Geometry: final body of the model. Coordinates: model frame, mm. A direction names the side the tool comes from. Give positions to 0.01 mm unless a question says otherwise; leave off trailing zeros. Write each loop counter-clockwise with the first axis right and the second up, starting at its lowest first coordinate (ties: lowest second). Pieces come first, ordered by that corner, then holes. Notation, with made-up numbers: (-33, 60) -> (-14, 60) arc R17 ccw to (-14, 92) -> close; hole circle Ø3 at (22, 38). An arc over 180 degrees is marked (long way). Answer in a Markdown table with one row per item. Add a question column.
from build123d import *

# Parameters (mm, degrees)
ESQUISSE3_R        = 2
ESQUISSE3_W        = 6
ESQUISSE3_H        = 6
ESQUISSE3_W_2      = 6.1
ESQUISSE3_H_2      = 6.1
ESQUISSE3_W_3      = 6.2
ESQUISSE3_H_3      = 6.2
ESQUISSE3_W_4      = 6.3
ESQUISSE3_H_4      = 6.3
BOSS_EXTRU_1_DEPTH = 6


with BuildPart() as part:
    # Esquisse3 → Boss.-Extru.1 (new body)
    with BuildSketch(Plane.XY):
        with BuildLine():
            Line((-87.161685907, 41.494801679), (-87.161685907, -2.505198321))
            Line((-87.161685907, -2.505198321), (-59.161685907, -2.505198321))
            Line((-59.161685907, -2.505198321), (-59.161685907, 41.494801679))
            ThreePointArc((-59.161685907, 41.494801679), (-73.161685907, 44.961803356), (-87.161685907, 41.494801679))
        make_face()
        with Locations((-73.161685907, 34.494801679)):
            Circle(ESQUISSE3_R, mode=Mode.SUBTRACT)
        with Locations((-73.161685907, 24.544801679)):
            Circle(ESQUISSE3_R, mode=Mode.SUBTRACT)
        with Locations((-73.161685907, 14.594801679)):
            Circle(ESQUISSE3_R, mode=Mode.SUBTRACT)
        with Locations((-73.161685907, 4.644801679)):
            Circle(ESQUISSE3_R, mode=Mode.SUBTRACT)
        with Locations((-80.161685907, 34.494801679)):
            Rectangle(ESQUISSE3_W, ESQUISSE3_H, mode=Mode.SUBTRACT)
        with Locations((-66.161685907, 34.494801679)):
            Rectangle(ESQUISSE3_W, ESQUISSE3_H, mode=Mode.SUBTRACT)
        with Locations((-80.161685907, 24.544801679)):
            Rectangle(ESQUISSE3_W_2, ESQUISSE3_H_2, mode=Mode.SUBTRACT)
        with Locations((-66.161685907, 24.544801679)):
            Rectangle(ESQUISSE3_W_2, ESQUISSE3_H_2, mode=Mode.SUBTRACT)
        with Locations((-80.161685907, 14.594801679)):
            Rectangle(ESQUISSE3_W_3, ESQUISSE3_H_3, mode=Mode.SUBTRACT)
        with Locations((-66.161685907, 14.594801679)):
            Rectangle(ESQUISSE3_W_3, ESQUISSE3_H_3, mode=Mode.SUBTRACT)
        with Locations((-80.161685907, 4.644801679)):
            Rectangle(ESQUISSE3_W_4, ESQUISSE3_H_4, mode=Mode.SUBTRACT)
        with Locations((-66.161685907, 4.644801679)):
            Rectangle(ESQUISSE3_W_4, ESQUISSE3_H_4, mode=Mode.SUBTRACT)
    extrude(amount=BOSS_EXTRU_1_DEPTH)


solid = part.part
Q1. Section B-B on y = 35. Return loops of the section in (x, z), and give its area (3 significant figures).
Q2. Section A-A on x = -66.5. Return loops of the section in (y, z), and give its area (3 significant figures).
Q3. Pull-direction query (Y, two-part tool) for faces 3 (the flat face through (-80, 17.695, 3)), 4 (the flat face through (-59.162, 19, 3)), 5 (the cylindrical face through (-72.96, 44.96, 2.96)); classes: +Y half, -Y half, draft (parallel to the pull), parting line (faces both ways), or undercut.
Q4. Contact query for flat-ended pins moving along their axis: pin 1 Ø1.5 at (x, z) = (-76, 1) entering from +Y; pin 2 Ø6 at (x, y) = (-68.5, 12.5) entering from +Z. Output: stop coordinate, or through.
Q5. Access query for faces 1 (the flat face through (-66, 21.495, 3)), 2 (the flat face through (-73, -2.505, 3)). Directions: +Z, -Z, +X, -X, +Y, -Y. A direction counts if a zero-diameter tool reaches every point of the face in a straight line with its end or side. Return the directions, or none.
Q6. Section C-C on x = -71.75. Return loops of the section in (y, z).
Q7. Section D-D on z = 3.55. Count the separate pieces of the cut face and the enclosed holes in it, and give its area (3 significant figures).
Q8. Line query: probe 1 along X at (y, z) = (4.5, 2); probe 2 along X at (y, z) = (24.5, 0.7); probe 3 along Y at (x, z) = (-68.5, 1.4). Output: solid intervals per line, ascending. Write a range as from..to.
Checks:
| question | item | result |
|---|---|---|
| 1 | outline | (-87.16, 0) -> (-83.16, 0) -> (-83.16, 6) -> (-87.16, 6) -> close; (-77.16, 0) -> (-75.1, 0) -> (-75.1, 6) -> (-77.16, 6) -> close; (-71.23, 0) -> (-69.16, 0) -> (-69.16, 6) -> (-71.23, 6) -> close; (-63.16, 0) -> (-59.16, 0) -> (-59.16, 6) -> (-63.16, 6) -> close |
| 1 | area | 72.8 mm^2 |
| 2 | outline | (-2.51, 0) -> (1.49, 0) -> (1.49, 6) -> (-2.51, 6) -> close; (7.79, 0) -> (11.49, 0) -> (11.49, 6) -> (7.79, 6) -> close; (17.69, 0) -> (21.49, 0) -> (21.49, 6) -> (17.69, 6) -> close; (27.59, 0) -> (31.49, 0) -> (31.49, 6) -> (27.59, 6) -> close; (37.49, 0) -> (44.21, 0) -> (44.21, 6) -> (37.49, 6) -> close |
| 2 | area | 133 mm^2 |
| 3 | face 3 | undercut |
| 3 | face 4 | draft |
| 3 | face 5 | +Y half |
| 4 | pin 1 | y = 44.89 |
| 4 | pin 2 | z = 6 |
| 5 | face 1 | +Z, -Z |
| 5 | face 2 | +Z, -Z, +X, -X, -Y |
| 6 | outline | (-2.51, 0) -> (3.23, 0) -> (3.23, 6) -> (-2.51, 6) -> close; (6.06, 0) -> (13.18, 0) -> (13.18, 6) -> (6.06, 6) -> close; (16.01, 0) -> (23.13, 0) -> (23.13, 6) -> (16.01, 6) -> close; (25.96, 0) -> (33.08, 0) -> (33.08, 6) -> (25.96, 6) -> close; (35.91, 0) -> (44.93, 0) -> (44.93, 6) -> (35.91, 6) -> close |
| 7 | separate pieces | 1 |
| 7 | enclosed holes | 12 |
| 7 | area | 945 mm^2 |
| 8 | probe 1 | -87.16..-83.31, -77.01..-75.16, -71.17..-69.31, -63.01..-59.16 |
| 8 | probe 2 | -87.16..-83.21, -77.11..-75.16, -71.16..-69.21, -63.11..-59.16 |
| 8 | probe 3 | -2.51..1.49, 7.79..11.49, 17.69..21.49, 27.59..31.49, 37.49..44.6 |
